Autodesk Inventor part; units mm, degrees
ref_plane "YZ Plane" through (0, 0, 0) normal (1, 0, 0) x (0, 1, 0)
ref_plane "XZ Plane" through (0, 0, 0) normal (0, 1, 0) x (-1, 0, 0)
ref_plane "XY Plane" through (0, 0, 0) normal (0, 0, 1) x (1, 0, 0)
sketch "Skizze1" plane through (0, 0, 0) normal (0, 0, 1) x (1, 0, 0)
  line L0 (0, 113.1371) -> (56.5685, 56.5685)
  line L1 (56.5685, 56.5685) -> (0, 0) construction
  line L2 (0, 0) -> (-56.5685, 56.5685) construction
  line L3 (-56.5685, 56.5685) -> (0, 113.1371)
  line L4 (0, 0) -> (-109.9706, 0) construction
  line L5 (-56.5685, 56.5685) -> (-56.5685, 0)
  line L6 (56.5685, 56.5685) -> (56.5685, 0)
  line L7 (-56.5685, 0) -> (56.5685, 0)
  dimension "d0" = 45
  dimension "d1" = 80
extrude "Extrusion1" add sketch "Skizze1" along normal blind 5
sketch "Skizze2" plane through (0, 0, 0) normal (0, 0, -1) x (-1, 0, 0)
  line L0 (-56.5685, 0) -> (56.5685, 0)
  line L1 (56.5685, 0) -> (56.5685, 5)
  line L2 (56.5685, 5) -> (-56.5685, 5)
  line L3 (-56.5685, 5) -> (-56.5685, 0)
  line L4 (56.5685, 0) -> (-56.5685, 0) construction
  line L5 (56.5685, 56.5685) -> (56.5685, 0) construction
  line L6 (0, 113.1371) -> (56.5685, 56.5685) construction
  line L7 (-56.5685, 56.5685) -> (0, 113.1371) construction
  line L8 (-56.5685, 0) -> (-56.5685, 56.5685) construction
  point P0 (0, 0)
  dimension "d4" = 5
extrude "Extrusion2" add sketch "Skizze2" along normal blind 55
sketch "Skizze3" plane through (56.5685, 0, 5) normal (1, 0, 0) x (0, 0, -1)
  line L0 (5, 5) -> (5, 56.5685) construction
  line L1 (5, 5) -> (60, 5) construction
  line L2 (5, 56.5685) -> (60, 5)
  line L3 (60, 5) -> (5, 5)
  line L4 (5, 5) -> (5, 56.5685)
  point P0 (5, 0)
extrude "Extrusion3" add sketch "Skizze3" against normal blind 5
sketch "Skizze4" plane through (-56.5685, 0, 5) normal (-1, 0, 0) x (0, 0, 1)
  line L0 (-5, 5) -> (-60, 5)
  line L1 (-5, 56.5685) -> (-5, 5)
  line L2 (-5, 56.5685) -> (-60, 5)
  point P0 (-5, 0)
extrude "Extrusion4" add sketch "Skizze4" against normal blind 5
sketch "Skizze5" plane through (51.5685, 5, 0) normal (0, 1, 0) x (1, 0, 0)
  line L0 (-15, 35) -> (-88.1371, 35) construction
  line L1 (-15, 38.1623) -> (-88.1371, 38.1623)
  line L2 (-88.1371, 31.8377) -> (-15, 31.8377)
  arc A0 (-15, 31.8377) -> (-15, 38.1623) centre (-15, 35) ccw
  arc A1 (-88.1371, 38.1623) -> (-88.1371, 31.8377) centre (-88.1371, 35) ccw
  line L3 (-103.1371, 55) -> (-103.1371, 0) construction
  line L4 (0, 0) -> (-103.1371, 0) construction
  line L5 (0, 0) -> (0, 55) construction
  line L6 (-103.1371, 55) -> (0, 55) construction
  point P0 (-51.5685, 0)
  point P1 (-51.5685, 35)
  dimension "d11" = 20
  dimension "d12" = 15
  dimension "d13" = 15
extrude "Extrusion5" cut sketch "Skizze5" against normal through all
sketch "Skizze6" plane through (0, 0, 5) normal (0, 0, 1) x (1, 0, 0)
  line L0 (-56.5685, 0) -> (56.5685, 0)
  line L1 (56.5685, 0) -> (56.5685, 56.5685)
  line L2 (56.5685, 56.5685) -> (0, 113.1371)
  line L3 (0, 113.1371) -> (-56.5685, 56.5685)
  line L4 (-56.5685, 56.5685) -> (-56.5685, 0)
  line L5 (-61.5685, 58.6396) -> (0, 120.2082)
  line L6 (0, 120.2082) -> (61.5685, 58.6396)
  line L7 (61.5685, 58.6396) -> (61.5685, -4)
  line L8 (-61.5685, 58.6396) -> (-61.5685, -4)
  line L9 (-61.5685, -4) -> (61.5685, -4)
  line L10 (56.5685, 56.5685) -> (0, 113.1371)
  line L11 (-56.5685, 0) -> (56.5685, 0)
  point P0 (0, 0)
  dimension "d16" = 5
  dimension "d17" = 5
  dimension "d18" = 5
  dimension "d19" = 5
  dimension "d20" = 4
extrude "Extrusion6" add sketch "Skizze6" against normal up to surface (5 mm away)
sketch "Skizze7" plane through (-56.5685, 0, 0) normal (0, -1, 0) x (1, 0, 0)
  line L0 (113.1371, 0) -> (0, 0)
  line L1 (0, 0) -> (0, -55)
  line L2 (113.1371, -55) -> (0, -55)
  line L3 (113.1371, -55) -> (113.1371, 0)
  line L4 (20, -31.8377) -> (93.1371, -31.8377)
  arc A0 (93.1371, -38.1623) -> (93.1371, -31.8377) centre (93.1371, -35) ccw
  line L5 (93.1371, -38.1623) -> (20, -38.1623)
  arc A1 (20, -31.8377) -> (20, -38.1623) centre (20, -35) ccw
  point P0 (56.5685, 0)
extrude "Extrusion7" add sketch "Skizze7" along normal blind 3.4
sketch "Skizze8" plane through (0, 0, -55) normal (0, 0, -1) x (-1, 0, 0)
  line L0 (56.5685, -3.4) -> (56.5685, 56.5685) construction
  line L1 (56.5685, -3.4) -> (-56.5685, -3.4) construction
  line L2 (-56.5685, -3.4) -> (-56.5685, 56.5685) construction
  line L3 (-56.5685, 56.5685) -> (-51.5685, 56.5685) construction
  line L4 (-51.5685, 56.5685) -> (-51.5685, 5) construction
  line L5 (-51.5685, 5) -> (51.5685, 5) construction
  line L6 (51.5685, 5) -> (51.5685, 56.5685) construction
  line L7 (51.5685, 56.5685) -> (56.5685, 56.5685) construction
  line L8 (0, 120.2082) -> (-61.5685, 58.6396) construction
  line L9 (-61.5685, 58.6396) -> (-61.5685, -4) construction
  line L10 (-61.5685, -4) -> (61.5685, -4) construction
  line L11 (61.5685, -4) -> (61.5685, 58.6396) construction
  line L12 (61.5685, 58.6396) -> (0, 120.2082) construction
  line L13 (96.047, 0) -> (96.047, 100) construction
  point P0 (0, 0)
  dimension "d25" = 96.047
properties part number "Halterung_ID6"
Here's how the part is built. I have some questions about the finished solid (model axes, mm). A direction names the side the tool comes from. Coordinates: 2 decimals unless noted, no trailing zeros. Order: outer loops, then holes, each group sorted by start corner. A loop starts at its lowest first (then second) coordinate and runs counter-clockwise, first axis right, second up.
Item 1: If we section it at C-C on y = 10: List the corners of the cut face in (x, z) for me.
Result sheet:
outline: (-61.57, 0) - (-56.57, 0) - (-56.57, -49.67) - (-51.57, -49.67) - (-51.57, 0) - (51.57, 0) - (51.57, -49.67) - (56.57, -49.67) - (56.57, 0) - (61.57, 0) - (61.57, 5) - (-61.57, 5) - close
Item 2: If we section it at D-D on x = 3: List the corners of the cut face in (y, z) for me, plus the area to 3 significant figures.
Result sheet:
outline: (-4, 0) - (-3.4, 0) - (-3.4, -31.84) - (5, -31.84) - (5, 0) - (117.21, 0) - (117.21, 5) - (-4, 5) - close; (-3.4, -55) - (5, -55) - (5, -38.16) - (-3.4, -38.16) - close
area: 1,010 mm2
Item 3: For P1, Ø5, axis at x = -34.5, z = -41, coming from the -Y side; P2, Ø1.5, axis at x = 48, y = 21, coming from the -Z side; P3, Ø3, axis at y = 39, z = -18, coming from the -X side, each with a flat end and sliding along its axis, tell me the tip position at first contact or that it passes through.
Result sheet:
P1: stops at y = -3.4
P2: stops at z = 0
P3: stops at x = -56.57
Item 4: I need wall thicknesses on line 1 (Y direction, x = -2, z = -12.5); line 2 (X direction, y = 11.5, z = -48); line 3 (Z direction, x = 14.5, y = 64). Which ranges of each line are inside material? Lowest first, please.
Result sheet:
line 1: y = -3.4 to 5
line 2: x = -56.57 to -51.57, 51.57 to 56.57
line 3: z = 0 to 5
Item 5: If we section it at A-A on x = 30: List the corners of the cut face in (y, z) for me, plus the area to 3 significant figures.
Result sheet:
outline: (-4, 0) - (-3.4, 0) - (-3.4, -31.84) - (5, -31.84) - (5, 0) - (90.21, 0) - (90.21, 5) - (-4, 5) - close; (-3.4, -55) - (5, -55) - (5, -38.16) - (-3.4, -38.16) - close
area: 880 mm2
Item 6: If we section it at B-B on z = -35: List the corners of the cut face in (x, y) for me.
Result sheet:
outline: (-56.57, -3.4) - (-39.73, -3.4) - (-39.73, 5) - (-51.57, 5) - (-51.57, 23.75) - (-56.57, 23.75) - close; (39.73, -3.4) - (56.57, -3.4) - (56.57, 23.75) - (51.57, 23.75) - (51.57, 5) - (39.73, 5) - close
Item 7: For faces 4 (the face through (-51.568, 20, -16)), 5 (the face through (-1, -3.4, -27)), 6 (the face through (-56.568, 20, -21)), which set-ups out of +Z, -Z, +X, -X, +Y, -Y let a thin tool reach every point of the face, with its end or its side?
Result sheet:
face 4: -Z, +Y
face 5: -Z, +X, -X, -Y
face 6: -Z, -X, +Y, -Y
Item 8: If we mould it in two halves opening along Z, with no side actions, what happens to faces 1 (the face through (1, 1, -38.162)), 2 (the face through (61.568, 28, 3)), 3 (the face through (1, 1, -55))? For each: +Z half, -Z half, draft (parallel to the pull), parting line (faces both ways), or undercut.
Result sheet:
face 1: undercut
face 2: draft
face 3: -Z half
